```python
from build123d import *

# Parameters (mm, degrees)
F0_R     = 6
F1_DEPTH = 32
F2_W     = 12
F2_H     = 15
F2_H_2   = 2.026334039
F3_DEPTH = 30.001


with BuildPart() as f1:
    # F0 (on Right) → F1 (new body)
    with BuildSketch(Plane.YZ):
        with BuildLine():
            Line((0, -46.4834831254), (0, 35.5165168746))
            ThreePointArc((0, 35.5165168746), (-25.3237080242, 46.3986606262), (-15.7894736842, 20.5373069054))
            ThreePointArc((-15.7894736842, 20.5373069054), (-13.0980949996, 19.29583972), (-12, 16.5428509136))
            Line((-12, 16.5428509136), (-12, -46.4834831254))
            Line((-12, -46.4834831254), (0, -46.4834831254))
        make_face()
        with Locations((-15, 35.5165168746)):
            Circle(F0_R, mode=Mode.SUBTRACT)
    extrude(amount=F1_DEPTH)

    # F2 (on Front) → F3 (cut, through all)
    with BuildSketch(Plane.XZ):
        Polygon((10, 16.5428509136), (22, 16.5428509136), (22, 35.5165168746), (10, 35.5165168746), (10, 20.5373069054), align=None)
        with Locations((16, 43.0165168746)):
            Rectangle(F2_W, F2_H)
        with Locations((16, 15.5296838941)):
            Rectangle(F2_W, F2_H_2)
        with BuildLine():
            Line((10, -5.4834831254), (10, -30.4834831254))
            ThreePointArc((10, -30.4834831254), (16, -36.4834831254), (22, -30.4834831254))
            Line((22, -30.4834831254), (22, -5.4834831254))
            ThreePointArc((22, -5.4834831254), (16, 0.5165168746), (10, -5.4834831254))
        make_face()
        with BuildLine():
            Line((16.0000000715, -46.4834831254), (32, -46.4834831254))
            Line((32, -46.4834831254), (32, -30.4834831254))
            ThreePointArc((32, -30.4834831254), (31.8046622717, -32.9760020276), (31.2234186903, -35.4076605573))
            ThreePointArc((31.2234186903, -35.4076605573), (25.4131068776, -43.4215439891), (16.0000000715, -46.4834831254))
        make_face()
        with BuildLine():
            Line((0, -46.4834831254), (16.0000000715, -46.4834831254))
            ThreePointArc((16.0000000715, -46.4834831254), (4.6862915263, -41.7971916497), (0, -30.4834831254))
            Line((0, -30.4834831254), (0, -46.4834831254))
        make_face()
    extrude(amount=F3_DEPTH, mode=Mode.SUBTRACT)


solid = f1.part
```
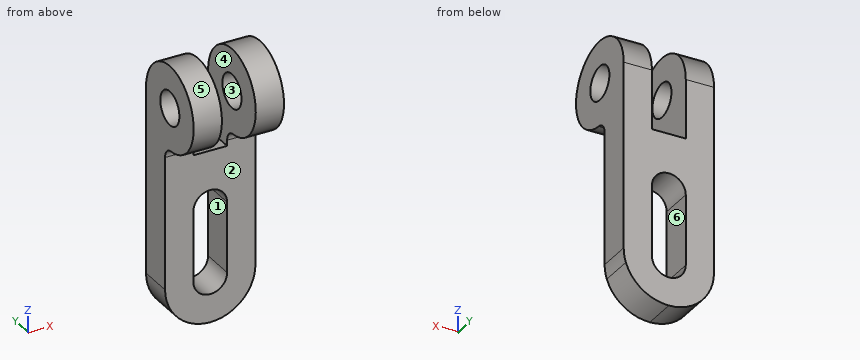
Input: part model. Units: mm. Frame: model coordinates. Face numbers are marked on the shaded views. A direction names the side the tool comes from. Round coordinates to 2 decimals unless told otherwise and drop trailing zeros. Loops run counter-clockwise (first coordinate to the right, second up) from the corner with the lowest first, then second, coordinate; pieces in that order, holes last. Notation, with made-up numbers: (50.5, -31.75) - (89.5, -31.75) arc R18 cw to (89.5, -14.75) - close; hole circle Ø2 at (-7.5, -34.5). An arc over 180 degrees is marked (long way). One line per item, written item: value. Start each with the question number.
(1) Draft query along Y for the marked faces 1, 2 and 3. Return one class per face: +Y half, -Y half, draft (parallel to the pull), parting line (faces both ways), or undercut.
(2) Section A-A, the plane z = -23.5. Return loops of the section in (x, y).
(3) Section D-D, the plane z = 36.5. Return loops of the section in (x, y).
(4) Section C-C, the plane y = -10.75. Return loops of the section in (x, z).
(5) Ray query, line 1 (X direction, y = -7, z = 32); line 2 (Y direction, x = 6, z = -33); line 3 (X direction, y = -3, z = -34.5). Return the intervals inside material, ascending. Write a range as [from, to].
(6) Section B-B, the plane x = 14. Return loops of the section in (y, z), plus the area to 3 significant figures.
(7) Access query for the marked faces 4, 5 and 6. Directions: +Z, -Z, +X, -X, +Y, -Y. A direction counts if a zero-diameter tool reaches every point of the face in a straight line with its end or side. Return the directions, or none.
(8) Contact query for flat-ended pins moving along their axis: P1, Ø1, axis at x = 12, z = -10, coming from the +Y side; P2, Ø6, axis at x = 14, y = -9, coming from the +Z side; P3, Ø2, axis at x = 3.5, y = -25.5, coming from the +Z side; P4, Ø4, axis at x = 8.5, y = -20, coming from the +Z side. Output: stop coordinate, or through.
Results below:
1. face 1: draft
1. face 2: -Y half
1. face 3: undercut
2. outline: (0, -12) - (10, -12) - (10, 0) - (0, 0) - close; (22, -12) - (32, -12) - (32, 0) - (22, 0) - close
3. outline: (0, -29.97) - (10, -29.97) - (10, -20.92) - (0, -20.92) - close; (0, -9.08) - (10, -9.08) - (10, -0.03) - (0, -0.03) - close; (22, -29.97) - (32, -29.97) - (32, -20.92) - (22, -20.92) - close; (22, -9.08) - (32, -9.08) - (32, -0.03) - (22, -0.03) - close
4. outline: (0, -30.48) arc R16 ccw to (32, -30.48) - (32, 31.28) - (22, 31.28) - (22, 14.52) - (10, 14.52) - (10, 31.28) - (0, 31.28) - close; (0, 39.75) - (10, 39.75) - (10, 49.9) - (0, 49.9) - close; (22, 39.75) - (32, 39.75) - (32, 49.9) - (22, 49.9) - close; hole (10, -30.48) arc R6 ccw to (22, -30.48) - (22, -5.48) arc R6 ccw to (10, -5.48) - close
5. line 1: [0, 10], [22, 32]
5. line 2: [-12, 0]
5. line 3: [0.51, 11.54], [20.46, 31.49]
6. outline: (-12, -46.36) - (0, -46.36) - (0, -36.14) - (-12, -36.14) - close; (-12, 0.17) - (0, 0.17) - (0, 14.52) - (-12, 14.52) - close
6. area: 295 mm^2
7. face 4: +Z, +Y, -Y
7. face 5: +X, -X
7. face 6: +Y, -Y
8. P1: through
8. P2: z = 14.52
8. P3: z = 47.12
8. P4: z = 50.21
